Here's how the part is built. I have some questions about the finished solid (model axes, mm). A direction names the side the tool comes from. Coordinates: 2 decimals unless noted, no trailing zeros. Write each loop counter-clockwise with the first axis right and the second up, starting at its lowest first coordinate (ties: lowest second). Pieces come first, ordered by that corner, then holes.
from build123d import *

# Parameters (mm, degrees)
SKETCH1_R           = 127.3
SKETCH1_R_2         = 125.3
BOSS_EXTRUDE1_DEPTH = 68
BOSS_EXTRUDE2_START = 2
SKETCH4_R           = 127.3
BOSS_EXTRUDE2_DEPTH = 2
SKETCH3_R           = 10
CUT_EXTRUDE3_DEPTH  = 193.443706055


with BuildPart() as part:
    # Sketch1 → Boss-Extrude1 (new body)
    with BuildSketch(Plane(origin=(0, 0, 0), x_dir=(1, 0, 0), z_dir=(0, 1, 0))):
        with Locations(Location((0, 0, 0), (0, 0, 270))):
            Circle(SKETCH1_R)
        with Locations(Location((0, 0, 0), (0, 0, 270))):
            Circle(SKETCH1_R_2, mode=Mode.SUBTRACT)
    extrude(amount=BOSS_EXTRUDE1_DEPTH)

    # Sketch4 → Boss-Extrude2 (add)
    with BuildSketch(Plane.XZ.offset(BOSS_EXTRUDE2_START)):
        with Locations(Location((0, 0, 0), (0, 0, 270))):
            Circle(SKETCH4_R)
    extrude(amount=-BOSS_EXTRUDE2_DEPTH)

    # Sketch3 → Cut-Extrude3 (cut, through all)
    with BuildSketch(Plane(origin=(0, 0, 0), x_dir=(0, 0, -1), z_dir=(1, 0, 0))):
        with Locations(Location((0, 10, 0), (0, 0, 270))):
            Circle(SKETCH3_R)
    extrude(amount=-CUT_EXTRUDE3_DEPTH, mode=Mode.SUBTRACT)


solid = part.part
1. On a 3-axis mill with a long thin cutter (end or side, diameter ignored), from which of +Z, -Z, +X, -X, +Y, -Y can I reach the whole of each face in a straight line? I mean faces 3 (the face through (-84, 68, 94)), 4 (the face through (-126.084, 0.763, 3.83)), 5 (the face through (-76.243, 33.524, -99.434)). Say none if no direction works.
2. If I drill on line 1 (Z direction, x = 0, y = 15); line 2 (Y direction, x = -125.5, z = 0); line 3 (Z direction, x = 34.5, y = 48.5), over which ranges is the centre line in solid material (lowest first)?
3. I want a section at B-B (y = 34). List the corners of the cut face in (x, z) for me, then the cut area to 3 significant figures.
4. Thinking about a two-plate mould opening in Z: for faces 1 (the face through (2, 0, 2)), 2 (the face through (2, -2, 2)), which applies, pulls with the +Z half, pulls with the -Z half, needs draft (parallel to the pull), parting line crosses it, or undercut?
5. For pin 1 Ø4 at (x, z) = (-6, -56.5) entering from +Y; pin 2 Ø1.5 at (y, z) = (34.5, -26.5) entering from +X; pin 3 Ø4 at (y, z) = (54, 56.5) entering from -X, each with a flat end and sliding along its axis, tell me the tip position at first contact or that it passes through.
6. I want a section at D-D (y = 10). List the corners of the cut face in (x, z) for me, then the cut area to 3 significant figures.
7. I want a section at A-A (x = 0). List the corners of the cut face in (y, z) for me, then the cut area to 3 significant figures.
8. I want a section at C-C (z = -35.5). List the corners of the cut face in (x, y) for me.
Response values:
1. face 3: +Z, -Z, +X, -X, +Y
1. face 4: -X
1. face 5: +Y
2. line 1: z = -127.3 to -125.3, 125.3 to 127.3
2. line 2: y = -2 to 0, 20 to 68
2. line 3: z = -122.54 to -120.46, 120.46 to 122.54
3. outline: circle Ø254.6 at (0, 0); hole circle Ø250.6 at (0, 0)
3. area: 1,590 mm2
4. face 1: undercut
4. face 2: needs draft
5. pin 1: stops at y = 0
5. pin 2: stops at x = 124.67
5. pin 3: stops at x = -115.04
6. outline: (-126.91, -10) arc R127.3 ccw (long way) to (-126.91, 10) - (-124.9, 10) arc R125.3 cw (long way) to (-124.9, -10) - close
6. area: 1,550 mm2
7. outline: (-2, -127.3) - (68, -127.3) - (68, -125.3) - (0, -125.3) - (0, 125.3) - (68, 125.3) - (68, 127.3) - (-2, 127.3) - close
7. area: 781 mm2
8. outline: (-122.25, -2) - (122.25, -2) - (122.25, 68) - (120.17, 68) - (120.17, 0) - (-120.17, 0) - (-120.17, 68) - (-122.25, 68) - close
